Could you check a few things on this model? Use its own coordinates, in mm. Round coordinates to 2 decimals unless told otherwise and drop trailing zeros. Loops run counter-clockwise (first coordinate to the right, second up) from the corner with the lowest first, then second, coordinate; pieces in that order, holes last. Notation, with made-up numbers: (53.5, 36) -> (97.5, 36) arc R8 cw to (97.5, 42) -> close; hole circle Ø11 at (18, 42.5). An arc over 180 degrees is marked (long way). One line per item, written item: value.
from build123d import *

# Parameters (mm, degrees)
SKETCH1_W              = 5.08
SKETCH1_H              = 5.08
BOSS_EXTRUDE1_DEPTH    = 241.3
SKETCH2_W              = 5.08
SKETCH2_H              = 5.08
BOSS_EXTRUDE2_DEPTH    = 116.84
FILLET1_R              = 2.54
LPATTERN1_COUNT        = 9
LPATTERN1_PITCH        = 29.5275
FILLET1_OF_LPATTERN1_R = 2.54


with BuildPart() as part:
    # Sketch1 → Boss-Extrude1 (new body)
    with BuildSketch(Plane(origin=(0, 0, 0), x_dir=(0, 0, -1), z_dir=(1, 0, 0))):
        Rectangle(SKETCH1_W, SKETCH1_H)
    extrude(amount=BOSS_EXTRUDE1_DEPTH)

    # Sketch2 → Boss-Extrude2 (add)
    with BuildSketch(Plane.XY):
        with Locations((2.54, 0)):
            Rectangle(SKETCH2_W, SKETCH2_H)
    boss_extrude2 = extrude(amount=BOSS_EXTRUDE2_DEPTH)

    # Fillet1
    fillet1_edges = [part.edges().sort_by_distance(p)[0] for p in [
        (2.54, -2.54, 116.84),
        (2.54, 2.54, 116.84),
    ]]
    fillet(fillet1_edges, radius=FILLET1_R - 0.0001)  # a hair under: the kernel refuses the full size

    # LPattern1: Boss-Extrude2 ×9, 3 skipped
    with Locations(*[(i * LPATTERN1_PITCH, 0, 0) for i in range(1, LPATTERN1_COUNT) if i not in (2, 4, 6)]):
        add(boss_extrude2)

    # Fillet1 of LPattern1
    fillet1_of_lpattern1_edges = [part.edges().sort_by_distance(p)[0] for p in [
        (32.0675, -2.54, 116.84),
        (32.0675, 2.54, 116.84),
        (91.1225, -2.54, 116.84),
        (91.1225, 2.54, 116.84),
        (150.1775, -2.54, 116.84),
        (150.1775, 2.54, 116.84),
        (209.2325, -2.54, 116.84),
        (209.2325, 2.54, 116.84),
        (238.76, -2.54, 116.84),
        (238.76, 2.54, 116.84),
    ]]
    fillet(fillet1_of_lpattern1_edges, radius=FILLET1_OF_LPATTERN1_R - 0.0001)  # a hair under: the kernel refuses the full size


solid = part.part
(1) I'm going to push flat-ended pins straight in: pin 1 Ø2.5 at (x, y) = (222.5, 1) entering from +Z; pin 2 Ø1.5 at (y, z) = (1.5, 19.5) entering from -X. Where does each tip first touch, or does it pass through?
Recorded:
pin 1: z = 2.54
pin 2: x = 0
(2) If we section it at A-A, the plane z = 13: Please give me the cut outline in (x, y).
Recorded:
outline: (0, -2.54) -> (5.08, -2.54) -> (5.08, 2.54) -> (0, 2.54) -> close; (29.53, -2.54) -> (34.61, -2.54) -> (34.61, 2.54) -> (29.53, 2.54) -> close; (88.58, -2.54) -> (93.66, -2.54) -> (93.66, 2.54) -> (88.58, 2.54) -> close; (147.64, -2.54) -> (152.72, -2.54) -> (152.72, 2.54) -> (147.64, 2.54) -> close; (206.69, -2.54) -> (211.77, -2.54) -> (211.77, 2.54) -> (206.69, 2.54) -> close; (236.22, -2.54) -> (241.3, -2.54) -> (241.3, 2.54) -> (236.22, 2.54) -> close
(3) If we section it at C-C, the plane x = 74: Please give me the cut outline in (y, z).
Recorded:
outline: (-2.54, -2.54) -> (2.54, -2.54) -> (2.54, 2.54) -> (-2.54, 2.54) -> close
(4) If we section it at B-B, the plane y = 1.75: Please give me the cut outline in (x, z).
Recorded:
outline: (0, -2.54) -> (241.3, -2.54) -> (241.3, 116.14) -> (236.22, 116.14) -> (236.22, 2.54) -> (211.77, 2.54) -> (211.77, 116.14) -> (206.69, 116.14) -> (206.69, 2.54) -> (152.72, 2.54) -> (152.72, 116.14) -> (147.64, 116.14) -> (147.64, 2.54) -> (93.66, 2.54) -> (93.66, 116.14) -> (88.58, 116.14) -> (88.58, 2.54) -> (34.61, 2.54) -> (34.61, 116.14) -> (29.53, 116.14) -> (29.53, 2.54) -> (5.08, 2.54) -> (5.08, 116.14) -> (0, 116.14) -> close
(5) If I drill on L1, parallel to X at y = 2.3, z = 31; L2, parallel to Z at x = 39, y = 2.25; L3, parallel to Z at x = 150, y = 0.95, over which ranges is the centre line in solid material (lowest first)?
Recorded:
L1: 0 to 5.08, 29.53 to 34.61, 88.58 to 93.66, 147.64 to 152.72, 206.69 to 211.77, 236.22 to 241.3
L2: -2.54 to 2.54
L3: -2.54 to 116.66
(6) Thinking about a two-plate mould opening in X: for faces 1 (the face through (17, 0, 2.54)), 2 (the face through (241.3, 0, 58)), 3 (the face through (119, 0, -2.54)), 4 (the face through (0, 0, 56)), which applies, released by +X, released by -X, zero draft, split by the parting line, or undercut?
Recorded:
face 1: undercut
face 2: released by +X
face 3: zero draft
face 4: released by -X
